For this review, take the finished solid that the model builds, in its own axes (mm). Face numbers are marked on the shaded views. A direction names the side the tool comes from. Give positions to 0.01 mm unless a question says otherwise; leave off trailing zeros. Write each loop counter-clockwise with the first axis right and the second up, starting at its lowest first coordinate (ties: lowest second). Pieces come first, ordered by that corner, then holes.
from build123d import *

# Parameters (mm, degrees)
SKETCH_1_R             = 13.7
SKETCH_1_R_2           = 12.2
EXTRUDE_1_DEPTH        = 10
SKETCH_3_W             = 9
SKETCH_3_H             = 55
EXTRUDE_2_DEPTH        = 3
SKETCH_4_W             = 24
SKETCH_4_H             = 35.5
EXTRUDE_3_DEPTH        = 4
FILLET_1_R             = 4
SKETCH_5_W             = 40
SKETCH_5_H             = 8
EXTRUDE_4_DEPTH        = 4
SKETCH_6_W             = 8
SKETCH_6_H             = 8
EXTRUDE_5_DEPTH        = 11
FILLET_2_R             = 6
HOLE_WIZARD_0_1_D      = 3.900000074
FILLET_2_OF_MIRROR_1_R = 6
SKETCH_11_W            = 8
SKETCH_11_H            = 8
EXTRUDE_6_DEPTH        = 11
HOLE_WIZARD_0_2_D      = 3.8999922
FILLET_3_R             = 3
FILLET_4_R             = 3
FILLET_5_R             = 3
SKETCH_14_W            = 10
SKETCH_14_H            = 3
EXTRUDE_7_DEPTH        = 30
FILLET_6_R             = 4
SKETCH_16_W            = 8
SKETCH_16_H            = 12.5
EXTRUDE_8_DEPTH        = 11
FILLET_7_R             = 4
FILLET_8_R             = 2
FILLET_9_R             = 2
FILLET_10_R            = 2
HOLE_WIZARD_0_3_D      = 3.900000074
HOLE_WIZARD_0_3_DEPTH  = 11
FILLET_11_R            = 5
FILLET_12_R            = 5
FILLET_13_R            = 3
FILLET_14_R            = 3
FILLET_15_R            = 3
FILLET_16_R            = 3
FILLET_17_R            = 3
FILLET_18_R            = 3
FILLET_19_R            = 3
FILLET_20_R            = 3


with BuildPart() as part:
    # ｽｹｯﾁ1 → ﾎﾞｽ - 押し出し1 (new body)
    with BuildSketch(Plane(origin=(0, 0, 0), x_dir=(1, 0, 0), z_dir=(0, 1, 0))):
        with Locations(Location((0, 0, 0), (0, 0, 270))):
            Circle(SKETCH_1_R)
        with Locations(Location((0, 0, 0), (0, 0, 270))):
            Circle(SKETCH_1_R_2, mode=Mode.SUBTRACT)
    extrude(amount=EXTRUDE_1_DEPTH)

    # ｽｹｯﾁ3 → ﾎﾞｽ - 押し出し2 (add)
    with BuildSketch(Plane.XY.offset(12.5)):
        with Locations((0, 27.5)):
            Rectangle(SKETCH_3_W, SKETCH_3_H)
    extrude(amount=EXTRUDE_2_DEPTH)

    # ｽｹｯﾁ4 → ﾎﾞｽ - 押し出し3 (add)
    with BuildSketch(Plane(origin=(0, 55, 0), x_dir=(1, 0, 0), z_dir=(0, 1, 0))):
        with Locations((0, 2.25)):
            Rectangle(SKETCH_4_W, SKETCH_4_H)
    extrude(amount=EXTRUDE_3_DEPTH)

    # ﾌｨﾚｯﾄ1
    fillet_1_edges = [part.edges().sort_by_distance(p)[0] for p in [
        (0, 55, 12.5),
    ]]
    fillet(fillet_1_edges, radius=FILLET_1_R)

    # ｽｹｯﾁ5 → ﾎﾞｽ - 押し出し4 (add)
    with BuildSketch(Plane(origin=(0, 55, 0), x_dir=(1, 0, 0), z_dir=(0, 1, 0))):
        with Locations((-20, 0)):
            Rectangle(SKETCH_5_W, SKETCH_5_H)
    extrude_4 = extrude(amount=EXTRUDE_4_DEPTH)

    # ｽｹｯﾁ6 → ﾎﾞｽ - 押し出し5 (add)
    with BuildSketch(Plane(origin=(0, 55, 0), x_dir=(1, 0, 0), z_dir=(0, 1, 0))):
        with Locations((-36, 0)):
            Rectangle(SKETCH_6_W, SKETCH_6_H)
    extrude_5 = extrude(amount=EXTRUDE_5_DEPTH)

    # ﾌｨﾚｯﾄ2
    fillet_2_edges = [part.edges().sort_by_distance(p)[0] for p in [
        (-32, 59, 0),
    ]]
    fillet(fillet_2_edges, radius=FILLET_2_R)

    # #0 すきま穴1 (through all)
    with Locations(Plane(origin=(0, 66, 0), x_dir=(1, 0, 0), z_dir=(0, 1, 0))):
        with Locations((-36, 0)):
            hole_wizard_0_1 = Hole(HOLE_WIZARD_0_1_D / 2)

    # ﾐﾗｰ1: ﾎﾞｽ - 押し出し4, ﾎﾞｽ - 押し出し5, #0 すきま穴1 across plane
    add(extrude_4.mirror(Plane(origin=(0, 0, 0), x_dir=(0, 0, 1), z_dir=(1, 0, 0))))
    add(extrude_5.mirror(Plane(origin=(0, 0, 0), x_dir=(0, 0, 1), z_dir=(1, 0, 0))))
    add(hole_wizard_0_1.mirror(Plane(origin=(0, 0, 0), x_dir=(0, 0, 1), z_dir=(1, 0, 0))), mode=Mode.SUBTRACT)

    # ﾌｨﾚｯﾄ2 of ﾐﾗｰ1
    fillet_2_of_mirror_1_edges = [part.edges().sort_by_distance(p)[0] for p in [
        (32, 59, 0),
    ]]
    fillet(fillet_2_of_mirror_1_edges, radius=FILLET_2_OF_MIRROR_1_R)

    # ｽｹｯﾁ11 → ﾎﾞｽ - 押し出し6 (add)
    with BuildSketch(Plane(origin=(0, 55, 0), x_dir=(1, 0, 0), z_dir=(0, 1, 0))):
        with Locations((0, 16)):
            Rectangle(SKETCH_11_W, SKETCH_11_H)
    extrude(amount=EXTRUDE_6_DEPTH)

    # #0 すきま穴2 (through all)
    with Locations(Plane(origin=(0, 66, 0), x_dir=(1, 0, 0), z_dir=(0, 1, 0))):
        with Locations((0, 16)):
            Hole(HOLE_WIZARD_0_2_D / 2)

    # ﾌｨﾚｯﾄ3
    fillet_3_edges = [part.edges().sort_by_distance(p)[0] for p in [
        (0, 59, -12),
    ]]
    fillet(fillet_3_edges, radius=FILLET_3_R)

    # ﾌｨﾚｯﾄ4
    fillet_4_edges = [part.edges().sort_by_distance(p)[0] for p in [
        (-4, 59, -14.5),
    ]]
    fillet(fillet_4_edges, radius=FILLET_4_R)

    # ﾌｨﾚｯﾄ5
    fillet_5_edges = [part.edges().sort_by_distance(p)[0] for p in [
        (4, 59, -14.5),
    ]]
    fillet(fillet_5_edges, radius=FILLET_5_R)

    # ｽｹｯﾁ14 → ﾎﾞｽ - 押し出し7 (add)
    with BuildSketch(Plane(origin=(0, 59, 0), x_dir=(1, 0, 0), z_dir=(0, 1, 0))):
        with Locations((0, -14)):
            Rectangle(SKETCH_14_W, SKETCH_14_H)
    extrude(amount=EXTRUDE_7_DEPTH)

    # ﾌｨﾚｯﾄ6
    fillet_6_edges = [part.edges().sort_by_distance(p)[0] for p in [
        (0, 59, 12.5),
    ]]
    fillet(fillet_6_edges, radius=FILLET_6_R)

    # ｽｹｯﾁ16 → ﾎﾞｽ - 押し出し8 (add)
    with BuildSketch(Plane(origin=(0, 89, 0), x_dir=(1, 0, 0), z_dir=(0, 1, 0))):
        with Locations((0, -9.25)):
            Rectangle(SKETCH_16_W, SKETCH_16_H)
    extrude(amount=EXTRUDE_8_DEPTH)

    # ﾌｨﾚｯﾄ7
    fillet_7_edges = [part.edges().sort_by_distance(p)[0] for p in [
        (0, 100, 15.5),
    ]]
    fillet(fillet_7_edges, radius=FILLET_7_R)

    # ﾌｨﾚｯﾄ8
    fillet_8_edges = [part.edges().sort_by_distance(p)[0] for p in [
        (0, 89, 12.5),
    ]]
    fillet(fillet_8_edges, radius=FILLET_8_R)

    # ﾌｨﾚｯﾄ9
    # the kernel refuses this fillet: 2 mm, written as the material it adds along each edge
    with BuildSketch(Plane(origin=(4, 89, 15.5), x_dir=(0, 1, 0), z_dir=(0, 0, -1))) as fillet_9_piece_1:
        with BuildLine():
            CenterArc((1.732050808, 2), FILLET_9_R, 210, 60)
            Line((0, 1), (0, 0))
            Line((0, 0), (1.732050808, 0))
        make_face()
    extrude(amount=3)

    # ﾌｨﾚｯﾄ10
    # the kernel refuses this fillet: 2 mm, written as the material it adds along each edge
    with BuildSketch(Plane(origin=(-4, 89, 12.5), x_dir=(-1, 0, 0), z_dir=(0, 0, 1))) as fillet_10_piece_1:
        with BuildLine():
            CenterArc((2, -1.732050808), FILLET_10_R, 120, 60)
            Line((0, -1.732050808), (0, 0))
            Line((0, 0), (1, 0))
        make_face()
    extrude(amount=3)

    # #0 すきま穴3
    with Locations(Plane(origin=(0, 100, 0), x_dir=(1, 0, 0), z_dir=(0, 1, 0))):
        with Locations((0, -7)):
            Hole(HOLE_WIZARD_0_3_D / 2, depth=HOLE_WIZARD_0_3_DEPTH)

    # ﾌｨﾚｯﾄ11
    fillet_11_edges = [part.edges().sort_by_distance(p)[0] for p in [
        (12, 57, -20),
    ]]
    fillet(fillet_11_edges, radius=FILLET_11_R)

    # ﾌｨﾚｯﾄ12
    fillet_12_edges = [part.edges().sort_by_distance(p)[0] for p in [
        (-12, 57, -20),
    ]]
    fillet(fillet_12_edges, radius=FILLET_12_R)

    # ﾌｨﾚｯﾄ13
    fillet_13_edges = [part.edges().sort_by_distance(p)[0] for p in [
        (-40, 60.5, -4),
    ]]
    fillet(fillet_13_edges, radius=FILLET_13_R)

    # ﾌｨﾚｯﾄ14
    fillet_14_edges = [part.edges().sort_by_distance(p)[0] for p in [
        (-40, 60.5, 4),
    ]]
    fillet(fillet_14_edges, radius=FILLET_14_R)

    # ﾌｨﾚｯﾄ15
    fillet_15_edges = [part.edges().sort_by_distance(p)[0] for p in [
        (40, 60.5, -4),
    ]]
    fillet(fillet_15_edges, radius=FILLET_15_R)

    # ﾌｨﾚｯﾄ16
    fillet_16_edges = [part.edges().sort_by_distance(p)[0] for p in [
        (40, 60.5, 4),
    ]]
    fillet(fillet_16_edges, radius=FILLET_16_R)

    # ﾌｨﾚｯﾄ17
    fillet_17_edges = [part.edges().sort_by_distance(p)[0] for p in [
        (4, 94.5, 3),
    ]]
    fillet(fillet_17_edges, radius=FILLET_17_R)

    # ﾌｨﾚｯﾄ18
    fillet_18_edges = [part.edges().sort_by_distance(p)[0] for p in [
        (-4, 94.5, 3),
    ]]
    fillet(fillet_18_edges, radius=FILLET_18_R)

    # ﾌｨﾚｯﾄ19
    fillet_19_edges = [part.edges().sort_by_distance(p)[0] for p in [
        (4.5, 5, 12.939860896),
    ]]
    fillet(fillet_19_edges, radius=FILLET_19_R)

    # ﾌｨﾚｯﾄ20
    fillet_20_edges = [part.edges().sort_by_distance(p)[0] for p in [
        (-4.5, 5, 12.939860896),
    ]]
    fillet(fillet_20_edges, radius=FILLET_20_R)


solid = part.part
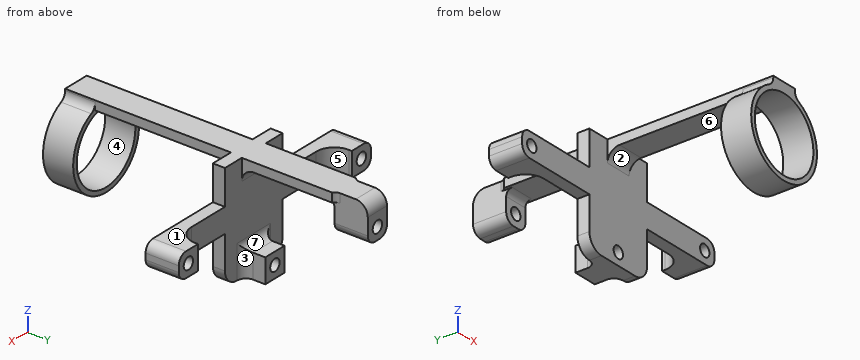
(1) The part is to be moulded in two halves that separate along Y. For the marked faces 1, 2 and 3, say which applies: +Y half, -Y half, draft (parallel to the pull), parting line (faces both ways), or undercut.
(2) We need section B-B (y = 19.5). Write out the cut boundary in (x, z), and give its area (3 significant figures).
(3) We need section A-A (y = 7.5). Write out the cut boundary in (x, z).
(4) For L1, parallel to X at y = 2, z = 0; L2, parallel to Z at x = 0, y = 95.5; L3, parallel to Z at x = -36, y = 63, list the stretches that pass through material, from the lowest coordinate up.
(5) Tool access review of the marked faces 4, 5, 6 and 7: name each direction out of +Z, -Z, +X, -X, +Y, -Y from which nothing blocks a thin tool from reaching the whole face with its end or side.
(6) Clearance check with flat-ended pins moving along their axes: pin 1 Ø5 at (x, y) = (0.5, 72.5) entering from -Z; pin 2 Ø2.5 at (x, z) = (0.5, -17.5) entering from +Y; pin 3 Ø12 at (x, y) = (-30, 61.5) entering from -Z; pin 4 Ø4 at (x, z) = (5, 11.5) entering from +Y. State where each tip first meets the part, or that it passes through.
(7) We need section C-C (x = -22). Write out the cut boundary in (y, z).
The answers:
1. face 1: draft
1. face 2: undercut
1. face 3: +Y half
2. outline: (-4.5, 12.5) - (4.5, 12.5) - (4.5, 15.5) - (-4.5, 15.5) - close
2. area: 27.0 mm2
3. outline: (-6.15, 12.24) arc R13.7 ccw (long way) to (6.15, 12.24) arc R3 cw to (4.5, 14.92) - (4.5, 15.5) - (-4.5, 15.5) - (-4.5, 14.92) arc R3 cw to start; hole circle Ø24.4 at (0, 0)
4. L1: x = -13.7 to -12.2, 12.2 to 13.7
4. L2: z = 3 to 5.05, 8.95 to 15.5
4. L3: z = -4 to -1.95, 1.95 to 4
5. face 4: -Y
5. face 5: +Z, -Z, +Y
5. face 6: -Z, +X, -X
5. face 7: +X, -X, +Y
6. pin 1: stops at z = 12.5
6. pin 2: stops at y = 66
6. pin 3: stops at z = -4
6. pin 4: stops at y = 100
7. outline: (55, -4) - (59, -4) - (59, 4) - (55, 4) - close
